The figure shows three views and two pictorial views of one solid part (mm, origin at its lowest corner). Answer the questions. A direction names the side the tool comes from. Round coordinates to 2 decimals unless told otherwise and drop trailing zeros. Loops run counter-clockwise (first coordinate to the right, second up) from the corner with the lowest first, then second, coordinate; pieces in that order, holes last. Notation, with made-up numbers: (16.5, -2.75) -> (33.5, -2.75) arc R28 cw to (33.5, 28.25) -> close; hole circle Ø9 at (25, 83.25). An arc over 180 degrees is marked (long way). Use a Markdown table: item, result. Add a question column.
Q1. Section C-C on x = 2.25 is taken. Give the vertices of the cut face in (y, z).
Q2. Section B-B on z = 30 is taken. Give the vertices of the cut face in (x, y), then the cut area to 3 significant figures.
Q3. Section D-D on y = 5 is taken. Give the vertices of the cut face in (x, z).
Q4. Given pin 1 Ø1.9 at (x, y) = (2, 3) entering from -Z; pin 2 Ø2 at (x, y) = (6.5, 6) entering from -Z; pin 3 Ø3 at (x, y) = (11, 20.5) entering from -Z, each flat-ended and moving along its own axis, determine where each tip first touches the part or whether it passes through.
Q5. Consider line 1 (Y direction, x = 3.45, z = 30); line 2 (Y direction, x = 7.05, z = 30); line 3 (X direction, y = 20.75, z = 40). Determine where each line is inside the solid, lowest interval first.
Q6. For a pull along Y with two mould halves and no side action, classify the marked faces 1, 2 and 3 as released by +Y, released by -Y, zero draft, split by the parting line, or undercut.
Q7. Section A-A on y = 20 is taken. Give the vertices of the cut face in (x, z).
Q8. Which of the six approach directions +Z, -Z, +X, -X, +Y, -Y give full straight-line access (tool end or side, diameter ignored) to the marked faces 4, 5, 6 and 7?
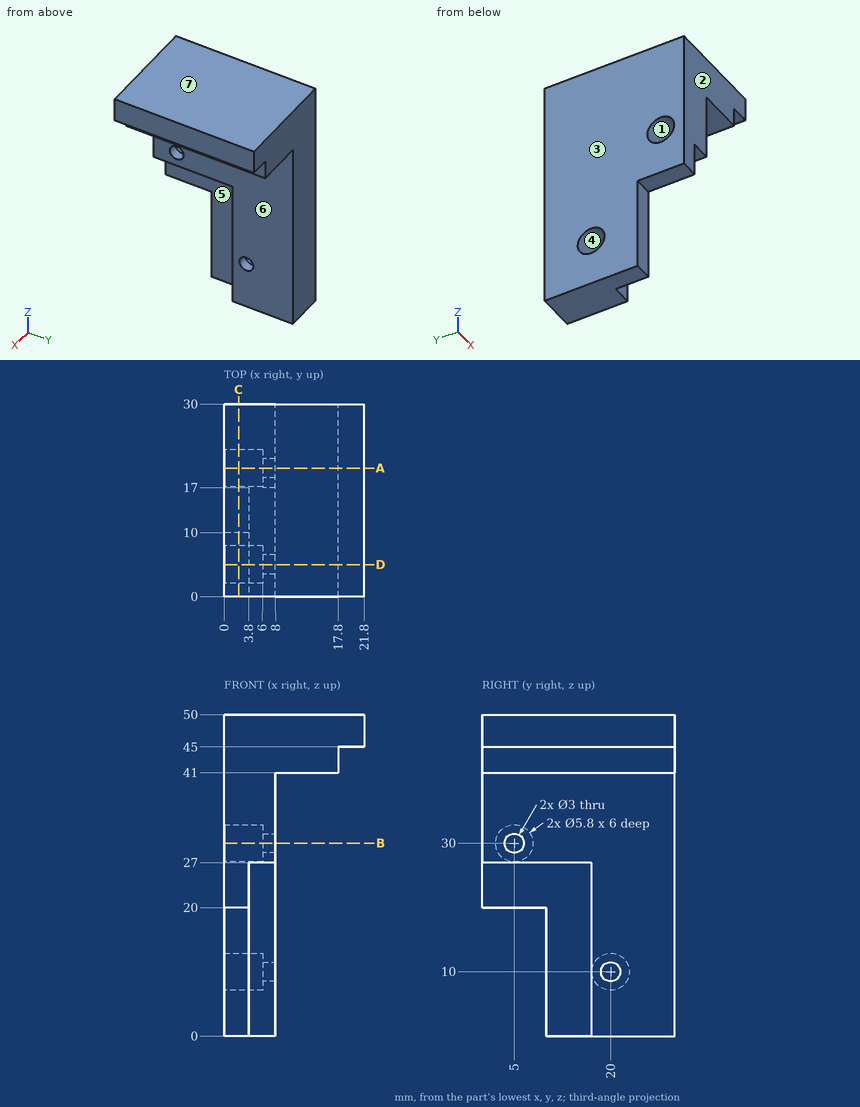
Checked values:
| question | item | result |
|---|---|---|
| 1 | outline | (0, 20) -> (10, 20) -> (10, 0) -> (30, 0) -> (30, 50) -> (0, 50) -> close; hole circle Ø5.8 at (5, 30); hole circle Ø5.8 at (20, 10) |
| 2 | outline | (0, 0) -> (8, 0) -> (8, 3.5) -> (6, 3.5) -> (6, 2.1) -> (0, 2.1) -> close; (0, 7.9) -> (6, 7.9) -> (6, 6.5) -> (8, 6.5) -> (8, 30) -> (0, 30) -> close |
| 2 | area | 199 mm2 |
| 3 | outline | (0, 20) -> (3.8, 20) -> (3.8, 27) -> (8, 27) -> (8, 28.5) -> (6, 28.5) -> (6, 27.1) -> (0, 27.1) -> close; (0, 32.9) -> (6, 32.9) -> (6, 31.5) -> (8, 31.5) -> (8, 41) -> (17.8, 41) -> (17.8, 45) -> (21.8, 45) -> (21.8, 50) -> (0, 50) -> close |
| 4 | pin 1 | stops at z = 20 |
| 4 | pin 2 | stops at z = 27 |
| 4 | pin 3 | stops at z = 41 |
| 5 | line 1 | y = 0 to 2.1, 7.9 to 30 |
| 5 | line 2 | y = 0 to 3.5, 6.5 to 30 |
| 5 | line 3 | x = 0 to 8 |
| 6 | face 1 | undercut |
| 6 | face 2 | released by -Y |
| 6 | face 3 | zero draft |
| 7 | outline | (0, 0) -> (8, 0) -> (8, 8.5) -> (6, 8.5) -> (6, 7.1) -> (0, 7.1) -> close; (0, 12.9) -> (6, 12.9) -> (6, 11.5) -> (8, 11.5) -> (8, 41) -> (17.8, 41) -> (17.8, 45) -> (21.8, 45) -> (21.8, 50) -> (0, 50) -> close |
| 8 | face 4 | -X |
| 8 | face 5 | -Z, +X, -Y |
| 8 | face 6 | -Z, +X, +Y, -Y |
| 8 | face 7 | +Z, +X, -X, +Y, -Y |
